```python
from build123d import *

# Parameters (mm, degrees)
F0_W     = 1600.2
F0_H     = 949.325
F1_DEPTH = 498.475
F2_W     = 45.155082
F2_H     = 923.191488
F2_W_2   = 53.135934
F2_H_2   = 919.007897
F2_W_3   = 1330.381736
F2_H_3   = 96.932329
F3_DEPTH = 508


with BuildPart() as f1:
    # F0 (on Front) → F1 (new body)
    with BuildSketch(Plane.XZ):
        with Locations((800.1, 474.6625)):
            Rectangle(F0_W, F0_H)
    extrude(amount=F1_DEPTH)

    # F2 (on face) → F3 (cut)
    with BuildSketch(Plane.XZ.offset(498.475)):
        with Locations((22.577541, 461.595744)):
            Rectangle(F2_W, F2_H)
        with Locations((1573.632033, 459.503948)):
            Rectangle(F2_W_2, F2_H_2)
        with Locations((802.38492, 48.466164)):
            Rectangle(F2_W_3, F2_H_3)
    extrude(amount=-F3_DEPTH, mode=Mode.SUBTRACT)


solid = f1.part
```
Verification items for the finished model (mm, model axes). A direction names the side the tool comes from. Round coordinates to 2 decimals unless told otherwise and drop trailing zeros. Write each loop counter-clockwise with the first axis right and the second up, starting at its lowest first coordinate (ties: lowest second). Pieces come first, ordered by that corner, then holes.
1. Draft check along X on faces 1 (the flat face through (1547.064, -253, 453)), 2 (the flat face through (137.194, -253, 48)), 3 (the flat face through (91, -246, 0)). Enter one of: +X half, -X half, draft (parallel to the pull), parting line (faces both ways), or undercut.
2. Section check A-A on y = -375. Enter the section's corners in (x, z) (3 decimals), plus the area to 3 significant figures.
3. Gauge pin test, flat ends, axial feed: P1, Ø2, axis at y = -218.5, z = 808.5, coming from the +X side; P2, Ø1.5, axis at y = -91, z = 490, coming from the -X side; P3, Ø6, axis at x = 195.5, y = -173, coming from the -Z side. Record the tip position at first contact, or that the pin passes through.
4. Scan lines: L1, parallel to X at y = -439.5, z = 223.5; L2, parallel to Z at x = 894.5, y = -104 (3 decimals); L3, parallel to X at y = -188, z = 88.5. Record each from-to range of solid material in increasing order.
5. Section check C-C on x = 728. Enter the section's corners in (y, z) (3 decimals), plus the area to 3 significant figures.
6. Access from +Z, -Z, +X, -X, +Y, -Y to the whole of each face (thin tool, end or side, straight path). Record for faces 4 (the flat face through (1600.2, -246, 934)), 5 (the flat face through (45.155, -253, 455)), 6 (the flat face through (1573, -253, 919.008)), 7 (the flat face through (1467.576, -253, 48)).
7. Section check B-B on z = 566. Enter the section's corners in (x, y) (3 decimals).
Answer:
1. face 1: +X half
1. face 2: undercut
1. face 3: draft
2. outline: (0, 923.191) - (45.155, 923.191) - (45.155, 0) - (137.194, 0) - (137.194, 96.932) - (1467.576, 96.932) - (1467.576, 0) - (1547.064, 0) - (1547.064, 919.008) - (1600.2, 919.008) - (1600.2, 949.325) - (0, 949.325) - close
2. area: 1,300,000 mm2
3. P1: stops at x = 1547.06
3. P2: stops at x = 45.16
3. P3: stops at z = 96.93
4. L1: x = 45.16 to 1547.06
4. L2: z = 96.932 to 949.325
4. L3: x = 45.16 to 137.19, 1467.58 to 1547.06
5. outline: (-498.475, 96.932) - (0, 96.932) - (0, 949.325) - (-498.475, 949.325) - close
5. area: 425,000 mm2
6. face 4: +Z, -Z, +X, +Y, -Y
6. face 5: -Z, -X, +Y, -Y
6. face 6: -Z, +X, +Y, -Y
6. face 7: -Z, +Y, -Y
7. outline: (45.155, -498.475) - (1547.064, -498.475) - (1547.064, 0) - (45.155, 0) - close
